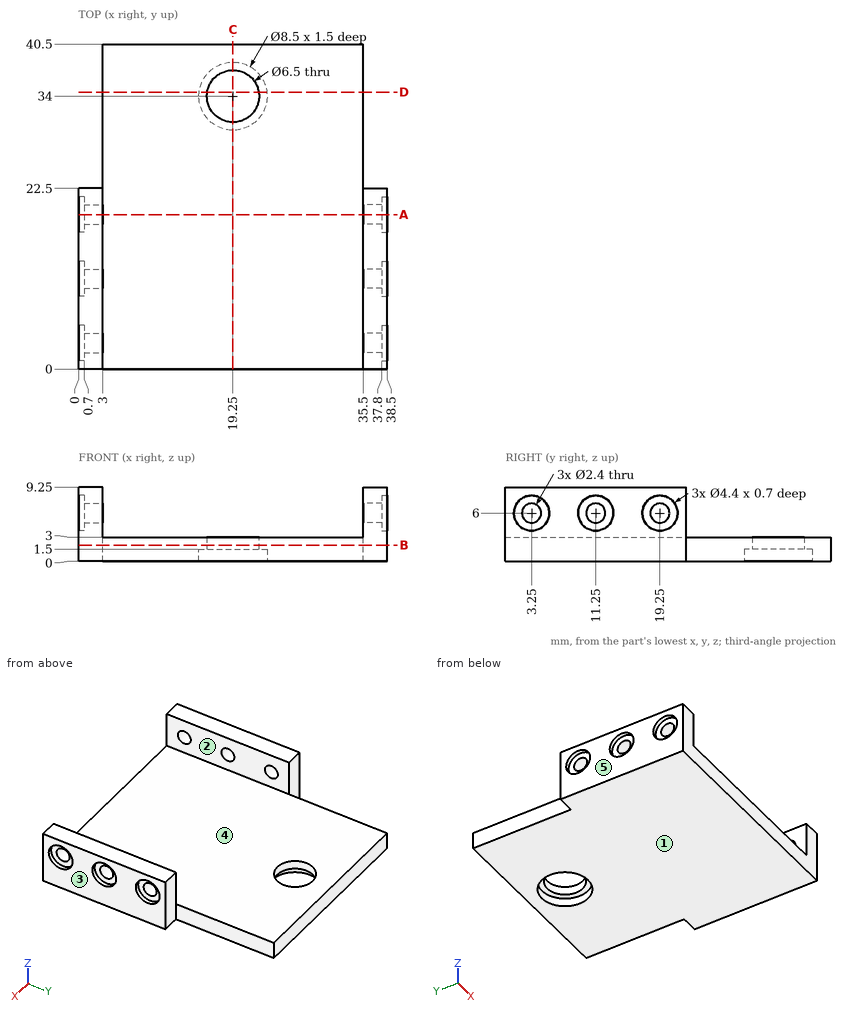
Study the drawing (mm; zero at the part's minimum x, y, z) and answer. A direction names the side the tool comes from. Give positions to 0.01 mm unless a question says otherwise; leave off trailing zeros. Write each loop counter-clockwise with the first axis right and the second up, starting at its lowest first coordinate (ties: lowest second). Pieces come first, ordered by that corner, then holes. Notation, with made-up numbers: (80.5, 35) - (138.5, 35) arc R29 cw to (138.5, 60) - close; hole circle Ø5 at (44, 12). An arc over 180 degrees is marked (long way). Write item = value, one per line. Start each with the question number.
Item 1: Each of these flat-tipped pins is pushed along its axis until it touches: P1, Ø2.5, axis at x = 36.5, z = 4, coming from the +Y side; P2, Ø1.5, axis at y = 31.5, z = 2, coming from the -X side; P3, Ø2.5, axis at y = 3.25, z = 6, coming from the -X side. Where does it stop, or does it pass through?
Item 2: Find section B-B (z = 2). Give the vertices of the cut face in (x, y).
Item 3: Find the intervals of material crossed by probe 1 along Y at (x, z) = (36.95, 6); probe 2 along Y at (x, z) = (38.3, 6); probe 3 along X at (y, z) = (7.5, 7.25), in increasing order. Write a range as [from, to].
Item 4: Find section C-C (x = 19.25). Give the vertices of the cut face in (y, z), then the cut area to 3 significant figures.
Item 5: A tool of negligible diameter and unlimited length cuts with its end or side. For the marked faces 1 and 2, from which of +Z, -Z, +X, -X, +Y, -Y can it reach the whole face along a straight path? Write none if from no direction.
Item 6: Find section D-D (y = 34.5). Give the vertices of the cut face in (x, z), then the cut area to 3 significant figures.
Item 7: The mould has two halves that part along X. Classify the marked faces 3, 4 and 5: +X half, -X half, draft (parallel to the pull), parting line (faces both ways), or undercut.
Item 8: Find section A-A (y = 19.25). Give the vertices of the cut face in (x, z), then the cut area to 3 significant figures.
Response:
q1.P1 = 22.5
q1.P2 = 3
q1.P3 = 0.7
q2.outline = (0, 0) - (38.5, 0) - (38.5, 22.5) - (35.5, 22.5) - (35.5, 40.5) - (3, 40.5) - (3, 22.5) - (0, 22.5) - close; hole circle Ø6.5 at (19.25, 34)
q3.probe_1 = [0, 2.05], [4.45, 10.05], [12.45, 18.05], [20.45, 22.5]
q3.probe_2 = [0, 1.05], [5.45, 9.05], [13.45, 17.05], [21.45, 22.5]
q3.probe_3 = [0, 3], [35.5, 38.5]
q4.outline = (0, 0) - (29.75, 0) - (29.75, 1.5) - (30.75, 1.5) - (30.75, 3) - (0, 3) - close; (37.25, 1.5) - (38.25, 1.5) - (38.25, 0) - (40.5, 0) - (40.5, 3) - (37.25, 3) - close
q4.area = 99.0 mm²
q5.face_1 = -Z, +X, -X, +Y, -Y
q5.face_2 = +Z, +Y, -Y
q6.outline = (3, 0) - (15.03, 0) - (15.03, 1.5) - (16.04, 1.5) - (16.04, 3) - (3, 3) - close; (22.46, 1.5) - (23.47, 1.5) - (23.47, 0) - (35.5, 0) - (35.5, 3) - (22.46, 3) - close
q6.area = 75.2 mm²
q7.face_3 = +X half
q7.face_4 = undercut
q7.face_5 = -X half
q8.outline = (0, 0) - (38.5, 0) - (38.5, 3.8) - (37.8, 3.8) - (37.8, 4.8) - (35.5, 4.8) - (35.5, 3) - (3, 3) - (3, 4.8) - (0.7, 4.8) - (0.7, 3.8) - (0, 3.8) - close; (0, 8.2) - (0.7, 8.2) - (0.7, 7.2) - (3, 7.2) - (3, 9.25) - (0, 9.25) - close; (35.5, 7.2) - (37.8, 7.2) - (37.8, 8.2) - (38.5, 8.2) - (38.5, 9.25) - (35.5, 9.25) - close
q8.area = 136 mm²
